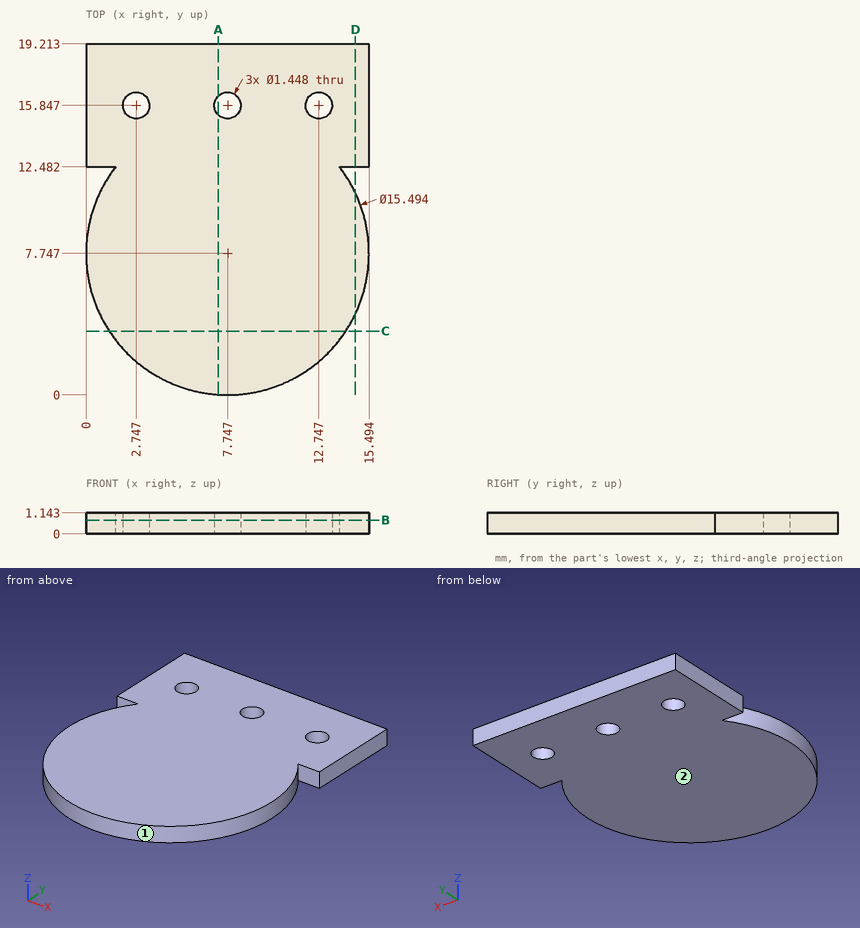
Job drawing, mm, ordinate dimensions from the low corner. One solid piece. Give positions to 0.01 mm unless a question says otherwise; leave off trailing zeros. Loops run counter-clockwise (first coordinate to the right, second up) from the corner with the lowest first, then second, coordinate; pieces in that order, holes last. Notation, with made-up numbers: (34, 41) - (76, 41) arc R22 cw to (76, 55) - close; hole circle Ø6 at (-1, -20.5). An arc over 180 degrees is marked (long way). Use one line per item in the form item = value.
(1) Cut at B-B (z = 0.75). Give the cut face in (x, y) (1 decimal).
Determined:
outline = (0, 12.5) - (1.6, 12.5) arc R7.7 ccw (long way) to (13.9, 12.5) - (15.5, 12.5) - (15.5, 19.2) - (0, 19.2) - close; hole circle Ø1.4 at (2.7, 15.8); hole circle Ø1.4 at (7.7, 15.8); hole circle Ø1.4 at (12.7, 15.8)
(2) Cut at D-D (x = 14.75). Give the cut face in (y, z) (1 decimal).
Determined:
outline = (4.4, 0) - (11.1, 0) - (11.1, 1.1) - (4.4, 1.1) - close; (12.5, 0) - (19.2, 0) - (19.2, 1.1) - (12.5, 1.1) - close
(3) Pull direction Y, two halves, no side cores. Call the marked faces 1 and 2: pulls with the +Y half, pulls with the -Y half, needs draft (parallel to the pull), parting line crosses it, or undercut.
Determined:
face_1 = undercut
face_2 = needs draft
(4) Cut at A-A (x = 7.25). Give the cut face in (y, z).
Determined:
outline = (0.02, 0) - (15.32, 0) - (15.32, 1.14) - (0.02, 1.14) - close; (16.37, 0) - (19.21, 0) - (19.21, 1.14) - (16.37, 1.14) - close
(5) Drill centre lines: L1, parallel to X at y = 7.5, z = 0.65 (1 decimal); L2, parallel to Y at x = 12.5, z = 0.8 (1 decimal); L3, parallel to X at y = 6, z = 0.35 (1 decimal). Where is each one in solid material? Low to high.
Determined:
L1 = 0 to 15.5
L2 = 1.6 to 15.2, 16.5 to 19.2
L3 = 0.2 to 15.3
(6) Cut at C-C (y = 3.5). Give the cut face in (x, z).
Determined:
outline = (1.27, 0) - (14.23, 0) - (14.23, 1.14) - (1.27, 1.14) - close
(7) Drop flat-ended pins along their axis: P1, Ø0.6, axis at x = 0.5, z = 1, coming from the -Y side; P2, Ø0.9, axis at x = 12.75, y = 15.85, coming from the +Z side. Give the stop position or say it passes through.
Determined:
P1 = 4.32
P2 = through
